Could you check a few things on this model? Use its own coordinates, in mm. Face numbers are marked on the shaded views. A direction names the side the tool comes from. Round coordinates to 2 decimals unless told otherwise and drop trailing zeros. Loops run counter-clockwise (first coordinate to the right, second up) from the corner with the lowest first, then second, coordinate; pieces in that order, holes last.
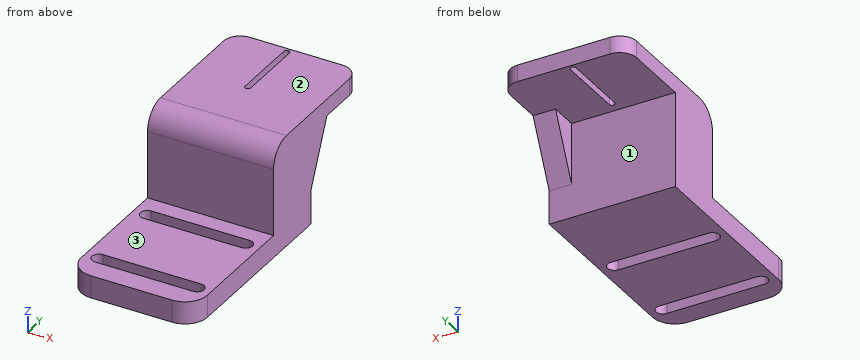
from build123d import *

# Parameters (mm, degrees)
SKETCH_1_W          = 45
SKETCH_1_H          = 72
EXTRUDE_1_DEPTH     = 8
SKETCH_3_W          = 45
SKETCH_3_H          = 23
EXTRUDE_2_DEPTH     = 32
SKETCH_4_W          = 45
SKETCH_4_H          = 6
EXTRUDE_3_DEPTH     = 30
CUT_EXTRUDE_1_DEPTH = 6
FILLET_1_R          = 8
RIB_1_REACH         = 133.568
SKETCH_7_WALL_W     = 289.301938088
SKETCH_7_WALL_H     = 8
FILLET_2_R          = 8
FILLET_3_R          = 6


with BuildPart() as part:
    # 草图1 → 凸台-拉伸1 (new body)
    with BuildSketch(Plane.XY):
        with Locations((49.020589592, -80.983410709)):
            Rectangle(SKETCH_1_W, SKETCH_1_H)
        with BuildLine():
            Line((31.520589592, -74.201396253), (66.520589592, -74.201396253))
            ThreePointArc((66.520589592, -74.201396253), (69.020589592, -76.701396253), (66.520589592, -79.201396253))
            Line((66.520589592, -79.201396253), (31.520589592, -79.201396253))
            ThreePointArc((31.520589592, -79.201396253), (29.020589592, -76.701396253), (31.520589592, -74.201396253))
        make_face(mode=Mode.SUBTRACT)
        with BuildLine():
            Line((31.520589592, -104.201396253), (66.520589592, -104.201396253))
            ThreePointArc((66.520589592, -104.201396253), (69.020589592, -106.701396253), (66.520589592, -109.201396253))
            Line((66.520589592, -109.201396253), (31.520589592, -109.201396253))
            ThreePointArc((31.520589592, -109.201396253), (29.020589592, -106.701396253), (31.520589592, -104.201396253))
        make_face(mode=Mode.SUBTRACT)
    extrude(amount=EXTRUDE_1_DEPTH)

    # 草图3 → 凸台-拉伸2 (add)
    with BuildSketch(Plane.XY.offset(8)):
        with Locations((49.020589592, -56.483410709)):
            Rectangle(SKETCH_3_W, SKETCH_3_H)
    extrude(amount=EXTRUDE_2_DEPTH)

    # 草图4 → 凸台-拉伸3 (add)
    with BuildSketch(Plane(origin=(0, -44.983410709, 0), x_dir=(1, 0, 0), z_dir=(0, 1, 0))):
        with Locations((49.020589592, -37)):
            Rectangle(SKETCH_4_W, SKETCH_4_H)
    extrude(amount=EXTRUDE_3_DEPTH)

    # 草图5 → 切除-拉伸1 (cut)
    with BuildSketch(Plane.XY.offset(40)):
        with BuildLine():
            Line((47.770589592, -16.983410709), (47.770589592, -40.983410709))
            ThreePointArc((47.770589592, -40.983410709), (46.770589592, -41.983410709), (45.770589592, -40.983410709))
            Line((45.770589592, -40.983410709), (45.770589592, -16.983410709))
            ThreePointArc((45.770589592, -16.983410709), (46.770589592, -15.983410709), (47.770589592, -16.983410709))
        make_face()
    extrude(amount=-CUT_EXTRUDE_1_DEPTH, mode=Mode.SUBTRACT)

    # 圆角1
    fillet_1_edges = [part.edges().sort_by_distance(p)[0] for p in [
        (71.520589592, -116.983410709, 4),
        (26.520589592, -116.983410709, 4),
    ]]
    fillet(fillet_1_edges, radius=FILLET_1_R)

    # 草图7 wall → 筋1 (add, up to next)
    with BuildSketch(Plane(origin=(71.520589592, -39.983410709, 23), x_dir=(0, -0.413802944301, -0.910366477463), z_dir=(0, 0.910366477463, -0.413802944301)), mode=Mode.PRIVATE) as rib_1_sk1:
        with Locations((0, 4)):
            Rectangle(SKETCH_7_WALL_W, SKETCH_7_WALL_H)
    rib_1_tool1 = extrude(rib_1_sk1.sketch, amount=-RIB_1_REACH, mode=Mode.PRIVATE) - part.part
    add(rib_1_tool1.solids().sort_by_distance((71.520589592, -39.983410709, 23))[0])

    # 圆角2
    fillet_2_edges = [part.edges().sort_by_distance(p)[0] for p in [
        (49.020589592, -67.983410709, 40),
    ]]
    fillet(fillet_2_edges, radius=FILLET_2_R)

    # 圆角3
    fillet_3_edges = [part.edges().sort_by_distance(p)[0] for p in [
        (26.520589592, -14.983410709, 37),
        (71.520589592, -14.983410709, 37),
    ]]
    fillet(fillet_3_edges, radius=FILLET_3_R)


solid = part.part
Item 1: Will these pins go through, and if not, where does the flat tip stop? pin 1 (8 mm diameter, centred on y = -40.5, z = 27.5, fed in from -X); pin 2 (3 mm diameter, centred on x = 47, z = 12, fed in from +Y); pin 3 (2 mm diameter, centred on x = 32.5, y = -31, fed in from -Z).
Results list:
pin 1: stops at x = 63.52
pin 2: stops at y = -44.98
pin 3: stops at z = 34
Item 2: If I drill on line 1 along Y through (x, z) = (42.5, 6.5); line 2 along X through (y, z) = (-33.5, 34.5); line 3 along Y through (x, z) = (64.5, 3), over which ranges is the centre line in solid material (lowest first)?
Results list:
line 1: y = -116.98 to -109.2, -104.2 to -79.2, -74.2 to -44.98
line 2: x = 26.52 to 45.77, 47.77 to 71.52
line 3: y = -116.92 to -109.2, -104.2 to -79.2, -74.2 to -44.98
Item 3: If we section it at A-A, the plane x = 44.5: Please give me the cut outline in (y, z).
Results list:
outline: (-116.98, 0) - (-109.2, 0) - (-109.2, 8) - (-116.98, 8) - close; (-104.2, 0) - (-79.2, 0) - (-79.2, 8) - (-104.2, 8) - close; (-74.2, 0) - (-44.98, 0) - (-44.98, 34) - (-14.98, 34) - (-14.98, 40) - (-59.98, 40) arc R8 ccw to (-67.98, 32) - (-67.98, 8) - (-74.2, 8) - close
Item 4: If we section it at B-B, the plane z = 3.5: Please give me the cut outline in (x, y).
Results list:
outline: (26.52, -108.98) arc R8 ccw to (34.52, -116.98) - (63.52, -116.98) arc R8 ccw to (71.52, -108.98) - (71.52, -44.98) - (26.52, -44.98) - close; hole (31.52, -109.2) - (66.52, -109.2) arc R2.5 ccw to (66.52, -104.2) - (31.52, -104.2) arc R2.5 ccw to start; hole (31.52, -79.2) - (66.52, -79.2) arc R2.5 ccw to (66.52, -74.2) - (31.52, -74.2) arc R2.5 ccw to start
Item 5: If we section it at C-C, the plane y = -38: Please give me the cut outline in (x, z).
Results list:
outline: (26.52, 34) - (45.77, 34) - (45.77, 40) - (26.52, 40) - close; (47.77, 34) - (63.52, 34) - (63.52, 27.36) - (71.52, 27.36) - (71.52, 40) - (47.77, 40) - close
Item 6: If we section it at D-D, the plane z = 35: Please give me the cut outline in (x, y).
Results list:
outline: (26.52, -67.4) - (71.52, -67.4) - (71.52, -20.98) arc R6 ccw to (65.52, -14.98) - (32.52, -14.98) arc R6 ccw to (26.52, -20.98) - close; hole (45.77, -40.98) arc R1 ccw to (47.77, -40.98) - (47.77, -16.98) arc R1 ccw to (45.77, -16.98) - close
Item 7: For the marked faces 1, 2 and 3, which set-ups out of +Z, -Z, +X, -X, +Y, -Y let a thin tool reach every point of the face, with its end or its side?
Results list:
face 1: -Z, -X, +Y
face 2: +Z, +X, -X, +Y, -Y
face 3: +Z, +X, -X, -Y
